```python
from build123d import *

# Parameters (mm, degrees)
F1_DEPTH = 5
F2_DEPTH = 5


with BuildPart() as f1:
    # F0 (on Top) → F1 (new body)
    with BuildSketch(Plane.XY):
        with BuildLine():
            ThreePointArc((35, 20), (33.535534, 23.535534), (30, 25))
            Line((30, 25), (-30, 25))
            ThreePointArc((-30, 25), (-33.535534, 23.535534), (-35, 20))
            Line((-35, 20), (-35, -20))
            ThreePointArc((-35, -20), (-33.535534, -23.535534), (-30, -25))
            Line((-30, -25), (30, -25))
            ThreePointArc((30, -25), (33.535534, -23.535534), (35, -20))
            Line((35, -20), (35, 20))
        make_face()
        with BuildLine():
            Line((-32, -19), (-32, 19))
            ThreePointArc((-32, 19), (-31.12132, 21.12132), (-29, 22))
            Line((-29, 22), (29, 22))
            ThreePointArc((29, 22), (31.12132, 21.12132), (32, 19))
            Line((32, 19), (32, -19))
            ThreePointArc((32, -19), (31.12132, -21.12132), (29, -22))
            Line((29, -22), (-29, -22))
            ThreePointArc((-29, -22), (-31.12132, -21.12132), (-32, -19))
        make_face(mode=Mode.SUBTRACT)
        with BuildLine():
            ThreePointArc((-29, 22), (-31.12132, 21.12132), (-32, 19))
            Line((-32, 19), (-32, -19))
            ThreePointArc((-32, -19), (-31.12132, -21.12132), (-29, -22))
            Line((-29, -22), (29, -22))
            ThreePointArc((29, -22), (31.12132, -21.12132), (32, -19))
            Line((32, -19), (32, 19))
            ThreePointArc((32, 19), (31.12132, 21.12132), (29, 22))
            Line((29, 22), (-29, 22))
        make_face()
    extrude(amount=F1_DEPTH)

    # F0 (on Top) → F2 (join)
    with BuildSketch(Plane.XY):
        with BuildLine():
            ThreePointArc((35, 20), (33.535534, 23.535534), (30, 25))
            Line((30, 25), (-30, 25))
            ThreePointArc((-30, 25), (-33.535534, 23.535534), (-35, 20))
            Line((-35, 20), (-35, -20))
            ThreePointArc((-35, -20), (-33.535534, -23.535534), (-30, -25))
            Line((-30, -25), (30, -25))
            ThreePointArc((30, -25), (33.535534, -23.535534), (35, -20))
            Line((35, -20), (35, 20))
        make_face()
        with BuildLine():
            Line((-32, -19), (-32, 19))
            ThreePointArc((-32, 19), (-31.12132, 21.12132), (-29, 22))
            Line((-29, 22), (29, 22))
            ThreePointArc((29, 22), (31.12132, 21.12132), (32, 19))
            Line((32, 19), (32, -19))
            ThreePointArc((32, -19), (31.12132, -21.12132), (29, -22))
            Line((29, -22), (-29, -22))
            ThreePointArc((-29, -22), (-31.12132, -21.12132), (-32, -19))
        make_face(mode=Mode.SUBTRACT)
    extrude(amount=-F2_DEPTH)


solid = f1.part
```
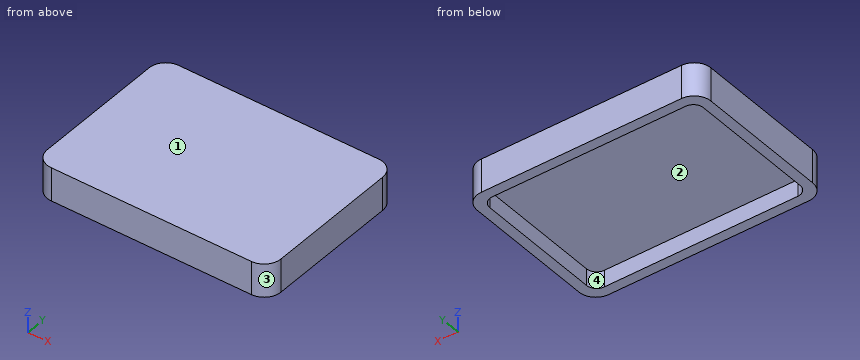
Design review of the part built by this model. Coordinates are the model's own, in mm. Face numbers are marked on the shaded views. Give positions to 0.01 mm unless a question says otherwise; leave off trailing zeros. Write each loop counter-clockwise with the first axis right and the second up, starting at its lowest first coordinate (ties: lowest second). Pieces come first, ordered by that corner, then holes. Notation, with made-up numbers: (10, 45.5) - (40, 45.5) arc R7 ccw to (40, 54.5) - close; hole circle Ø6 at (41, 42). An arc over 180 degrees is marked (long way). Return JSON: item names as keys, results as strings. Group by question number.
(1) We need section C-C, the plane y = -5. Give the boundary of the cut face in (x, z), then the cut area to 3 significant figures.
(2) Mouldability with a two-part tool opening along X and no side actions: class the marked faces 1, 2, 3 and 4 as +X half, -X half, draft (parallel to the pull), parting line (faces both ways), or undercut.
(3) We need section A-A, the plane z = -4. Give the boundary of the cut face in (x, y).
(4) Insertion check: pin 1 (10 mm diameter, centred on x = 1, y = -9, fed in from -Z). The pin has a flat end and moves straight along its axis. Give the tip position at first contact, or say it passes through.
(5) We need section B-B, the plane x = -25.5. Give the boundary of the cut face in (y, z), then the cut area to 3 significant figures.
(6) To check wall thickness, follow probe 1 along X at (y, z) = (2, -3.75); probe 2 along Y at (x, z) = (12, -2.5); probe 3 along Z at (x, y) = (13, -11.5). State the ranges of each line that lie inside material, in increasing order.
Reported:
{
 "1": {"outline": "(-35, -5) - (-32, -5) - (-32, 0) - (32, 0) - (32, -5) - (35, -5) - (35, 5) - (-35, 5) - close", "area": "380 mm2"},
 "2": {"face 1": "draft", "face 2": "undercut", "face 3": "+X half", "face 4": "undercut"},
 "3": {"outline": "(-35, -20) arc R5 ccw to (-30, -25) - (30, -25) arc R5 ccw to (35, -20) - (35, 20) arc R5 ccw to (30, 25) - (-30, 25) arc R5 ccw to (-35, 20) - close; hole (-32, -19) arc R3 ccw to (-29, -22) - (29, -22) arc R3 ccw to (32, -19) - (32, 19) arc R3 ccw to (29, 22) - (-29, 22) arc R3 ccw to (-32, 19) - close"},
 "4": {"pin 1": "stops at z = 0"},
 "5": {"outline": "(-25, -5) - (-22, -5) - (-22, 0) - (22, 0) - (22, -5) - (25, -5) - (25, 5) - (-25, 5) - close", "area": "280 mm2"},
 "6": {"probe 1": "x = -35 to -32, 32 to 35", "probe 2": "y = -25 to -22, 22 to 25", "probe 3": "z = 0 to 5"}
}
